from build123d import *

# Parameters (mm, degrees)
BOSS_EXTRUDE1_DEPTH = 4
FILLET1_R           = 20
SKETCH1_R           = 2.75
CUT_EXTRUDE3_DEPTH  = 131.855321132
BOSS_EXTRUDE2_START = 20
BOSS_EXTRUDE2_DEPTH = 20
SKETCH7_W           = 10
SKETCH7_H           = 20
BOSS_EXTRUDE3_DEPTH = 20
SKETCH8_W           = 12.2
SKETCH8_H           = 12.2
CUT_EXTRUDE4_DEPTH  = 3.1
CUT_EXTRUDE5_REACH  = 88.267
SKETCH8_3_W         = 12.2
SKETCH8_3_H         = 3.5


with BuildPart() as part:
    # Sketch3 → Boss-Extrude1 (new body)
    with BuildSketch(Plane(origin=(0, 0, 0), x_dir=(1, 0, 0), z_dir=(0, 1, 0))):
        with BuildLine():
            Line((22.912878475, 10), (44, 10))
            Line((44, 10), (54, 10))
            Line((54, 10), (54, -25))
            Line((54, -25), (44, -25))
            Line((44, -25), (44, -10))
            Line((44, -10), (22.912878475, -10))
            ThreePointArc((22.912878475, -10), (-25, 0), (22.912878475, 10))
        make_face()
    extrude(amount=BOSS_EXTRUDE1_DEPTH)

    # Fillet1
    fillet1_edges = [part.edges().sort_by_distance(p)[0] for p in [
        (22.912878475, 2, 10),
        (22.912878475, 2, -10),
    ]]
    fillet(fillet1_edges, radius=FILLET1_R)

    # Sketch1 → Cut-Extrude3 (cut, through all)
    with BuildSketch(Plane(origin=(103.38268991, 0, 0), x_dir=(1, 0, 0), z_dir=(0, 1, 0))):
        with Locations(Location((-66.469811435, 0, 0), (0, 0, 270))):
            Circle(SKETCH1_R)
        with BuildLine():
            ThreePointArc((-91.90785331, -6.625), (-92.397942073, -7.409305971), (-92.941547424, -8.157514548))
            ThreePointArc((-92.941547424, -8.157514548), (-92.639936187, -10.613940949), (-90.183509787, -10.312329712))
            ThreePointArc((-90.183509787, -10.312329712), (-89.496310569, -9.366481133), (-88.876764396, -8.375))
            ThreePointArc((-88.876764396, -8.375), (-89.517308853, -5.984455543), (-91.90785331, -6.625))
        make_face()
        with BuildLine():
            ThreePointArc((-91.13268991, 0), (-91.162530294, -0.854516803), (-91.251906068, -1.704870487))
            ThreePointArc((-91.251906068, -1.704870487), (-89.762489874, -3.681392534), (-87.785967827, -2.19197634))
            ThreePointArc((-87.785967827, -2.19197634), (-87.671056118, -1.098664461), (-87.63268991, 0))
            ThreePointArc((-87.63268991, 0), (-89.38268991, 1.75), (-91.13268991, 0))
        make_face()
        with BuildLine():
            ThreePointArc((-114.85752651, -6.625), (-115.498070966, -9.015544457), (-117.888615423, -8.375))
            ThreePointArc((-117.888615423, -8.375), (-118.437490185, -7.342716709), (-118.913019474, -6.27466044))
            ThreePointArc((-118.913019474, -6.27466044), (-117.946009267, -3.996527156), (-115.667875983, -4.963537363))
            ThreePointArc((-115.667875983, -4.963537363), (-115.291711023, -5.808417695), (-114.85752651, -6.625))
        make_face()
        with BuildLine():
            ThreePointArc((-111.25768991, -13.63990011), (-108.867145453, -12.999355653), (-109.50768991, -10.608811196))
            ThreePointArc((-109.50768991, -10.608811196), (-110.232802977, -10.155710264), (-110.924542982, -9.653131732))
            ThreePointArc((-110.924542982, -9.653131732), (-113.380969383, -9.954742969), (-113.079358146, -12.411169369))
            ThreePointArc((-113.079358146, -12.411169369), (-112.189978139, -13.057341768), (-111.25768991, -13.63990011))
        make_face()
        with BuildLine():
            ThreePointArc((-103.38268991, 13.25), (-105.13268991, 15), (-103.38268991, 16.75))
            ThreePointArc((-103.38268991, 16.75), (-102.214268974, 16.709197842), (-101.051540469, 16.586990151))
            ThreePointArc((-101.051540469, 16.586990151), (-99.562124275, 14.610468104), (-101.538646322, 13.121051911))
            ThreePointArc((-101.538646322, 13.121051911), (-102.458416633, 13.217723666), (-103.38268991, 13.25))
        make_face()
        with BuildLine():
            ThreePointArc((-111.25768991, 13.63990011), (-111.898234366, 11.249355653), (-109.50768991, 10.608811196))
            ThreePointArc((-109.50768991, 10.608811196), (-108.752736458, 11.010227067), (-107.971620679, 11.358002218))
            ThreePointArc((-107.971620679, 11.358002218), (-107.004610472, 13.636135502), (-109.282743756, 14.603145709))
            ThreePointArc((-109.282743756, 14.603145709), (-110.287035472, 14.156006229), (-111.25768991, 13.63990011))
        make_face()
    extrude(amount=CUT_EXTRUDE3_DEPTH, mode=Mode.SUBTRACT)

    # Sketch4 → Boss-Extrude2 (add)
    with BuildSketch(Plane.XZ.offset(BOSS_EXTRUDE2_START)):
        with BuildLine():
            Line((18.633899812, 16.666666667), (17.452315988, 15.609825965))
            ThreePointArc((17.452315988, 15.609825965), (16.092851842, 15.100708662), (14.747154343, 15.645173018))
            ThreePointArc((14.747154343, 15.645173018), (-21.5, 0), (14.747154343, -15.645173018))
            ThreePointArc((14.747154343, -15.645173018), (16.092851842, -15.100708662), (17.452315988, -15.609825965))
            Line((17.452315988, -15.609825965), (18.633899812, -16.666666667))
            ThreePointArc((18.633899812, -16.666666667), (-25, 0), (18.633899812, 16.666666667))
        make_face()
    extrude(amount=-BOSS_EXTRUDE2_DEPTH)

    # Sketch7 → Boss-Extrude3 (add)
    with BuildSketch(Plane(origin=(0, 4, 0), x_dir=(1, 0, 0), z_dir=(0, 1, 0))):
        with Locations((49, -15)):
            Rectangle(SKETCH7_W, SKETCH7_H)
    extrude(amount=BOSS_EXTRUDE3_DEPTH)

    # Sketch8 → Cut-Extrude4 (cut)
    with BuildSketch(Plane(origin=(54, 0, 0), x_dir=(0, 0, -1), z_dir=(1, 0, 0))):
        with Locations((-15, 14)):
            Rectangle(SKETCH8_W, SKETCH8_H)
    extrude(amount=-CUT_EXTRUDE4_DEPTH, mode=Mode.SUBTRACT)

    # Sketch8_3 → Cut-Extrude5 (cut, up to next)
    with BuildSketch(Plane(origin=(54, 0, 0), x_dir=(0, 0, -1), z_dir=(1, 0, 0)), mode=Mode.PRIVATE) as cut_extrude5_sk1:
        with Locations((-15, 20.1)):
            Rectangle(SKETCH8_3_W, SKETCH8_3_H)
    cut_extrude5_tool1 = extrude(cut_extrude5_sk1.sketch, amount=-CUT_EXTRUDE5_REACH, mode=Mode.PRIVATE) & part.part
    add(cut_extrude5_tool1.solids().sort_by_distance((54, 20.1, 15))[0], mode=Mode.SUBTRACT)


solid = part.part
Could you check a few things on this model? Use its own coordinates, in mm. A direction names the side the tool comes from. Give positions to 0.01 mm unless a question says otherwise; leave off trailing zeros. Order: outer loops, then holes, each group sorted by start corner. A loop starts at its lowest first (then second) coordinate and runs counter-clockwise, first axis right, second up.
1. Which directions (+Z, -Z, +X, -X, +Y, -Y) give clear straight access to the entire face, cutting with the end or side of a thin tool? Please do faces 4 (the cylindrical face through (15.71, 1.97, 1.11)), 5 (the flat face through (51.3, 16.3, 21.1)), 6 (the flat face through (44, 2, -10)), 7 (the cylindrical face through (16.1, -10.1, 15.1)).
Answers below:
face 4: +Y, -Y
face 5: +X
face 6: -Z, +X, +Y, -Y
face 7: -Y
2. Suppose I cut it at B-B (x = 7). Write out the boundary of the cut face in (y, z).
Answers below:
outline: (-20, -24) - (4, -24) - (4, 24) - (-20, 24) - (-20, 20.33) - (0, 20.33) - (0, -20.33) - (-20, -20.33) - close
3. Suppose I cut it at A-A (y = 20). Write out the boundary of the cut face in (x, z), plus the area to 3 significant figures.
Answers below:
outline: (44, 5) - (54, 5) - (54, 8.9) - (44, 8.9) - close; (44, 21.1) - (54, 21.1) - (54, 25) - (44, 25) - close
area: 78.0 mm2
4. Thinking about a two-plate mould opening in Y: for faces 1 (the cylindrical face through (0.937, 1.972, -13.217)), 2 (the flat face through (50.9, 13, 15)), 3 (the flat face through (47, 18.35, 15)), which applies, +Y half, -Y half, draft (parallel to the pull), parting line (faces both ways), or undercut?
Answers below:
face 1: draft
face 2: undercut
face 3: undercut
5. For pin 1 (14 mm diameter, centred on x = 26.5, z = -1, fed in from -Y); pin 2 (15 mm diameter, centred on x = -1, z = 11, fed in from +Y); pin 3 (1.5 mm diameter, centred on y = -2, z = 15.5, fed in from -X); pin 4 (1 mm diameter, centred on y = 6, z = -9, fed in from -X), each with a flat end and sliding along its axis, tell me the tip position at first contact or that it passes through.
Answers below:
pin 1: stops at y = 0
pin 2: stops at y = 4
pin 3: stops at x = -20.19
pin 4: passes through
6. Suppose I cut it at D-D (y = -6.5). Write out the boundary of the cut face in (x, z), plus the area to 3 significant figures.
Answers below:
outline: (14.75, -15.65) arc R21.5 cw (long way) to (14.75, 15.65) arc R2 ccw to (17.45, 15.61) - (18.63, 16.67) arc R25 ccw (long way) to (18.63, -16.67) - (17.45, -15.61) arc R2 ccw to start
area: 391 mm2
7. Suppose I cut it at C-C (y = 13.5). Write out the boundary of the cut face in (x, z), plus the area to 3 significant figures.
Answers below:
outline: (44, 5) - (54, 5) - (54, 8.9) - (50.9, 8.9) - (50.9, 21.1) - (54, 21.1) - (54, 25) - (44, 25) - close
area: 162 mm2
8. I need wall thicknesses on L1, parallel to X at y = 1, z = 0; L2, parallel to Z at x = 0, y = -11; L3, parallel to Y at x = -4, z = -9. Which ranges of each line are inside material? Lowest first, please.
Answers below:
L1: x = -25 to 12.25, 15.75 to 34.16, 39.66 to 54
L2: z = -25 to -21.5, 21.5 to 25
L3: y = 0 to 4
